Build history of the part. All positions in model axes, mm. A direction names the side the tool comes from. Give positions to 0.01 mm unless a question says otherwise; leave off trailing zeros. Write each loop counter-clockwise with the first axis right and the second up, starting at its lowest first coordinate (ties: lowest second). Pieces come first, ordered by that corner, then holes. Notation, with made-up numbers: (61, -17.5) -> (70, -17.5) arc R13 ccw to (70, -13.5) -> close; hole circle Ø5 at (18.25, 74). An arc over 180 degrees is marked (long way). One line per question, with ' | ' between items. Start each with the question number.
(1) Band-saw the part on B-B, the plane z = -41.5. Give the cut face in (x, y), and give its area (3 significant figures).
(2) Band-saw the part on C-C, the plane z = 10. Give the cut face in (x, y), and give its area (3 significant figures).
(3) Pin check, flat tips, straight feed: P1, Ø16, axis at x = -3, z = -45.5, coming from the -Y side; P2, Ø5, axis at y = -23.5, z = -55.5, coming from the +X side; P3, Ø7.5, axis at x = 17, y = -2, coming from the +Z side. Stop position of each tip, or through.
(4) Pull direction Y, two halves, no side cores. Call faces 6 (the flat face through (-16.26, 24.39, -4.52)), 7 (the cylindrical face through (-21.63, -19.44, -57.82)), 8 (the flat face through (-18.6, -20.2, -6)): released by +Y, released by -Y, zero draft, split by the parting line, or undercut.
(5) Tool access for faces 1 (the flat face through (-24.31, -16.18, -4.52)), 2 (the flat face through (16.26, -24.39, -4.52)), 3 (the flat face through (-24.11, 24.13, -50.4)), 4 (the flat face through (18, 17, -61)), 5 (the flat face through (-18, 0, 0)): list every direction of +Z, -Z, +X, -X, +Y, -Y with a clear straight run to the whole face (end or side of a thin tool).
(6) Drill centre lines: probe 1 along Y at (x, z) = (-20, -3.5); probe 2 along X at (y, z) = (0, -4.5); probe 3 along X at (y, z) = (11.5, -37.5). Where is each one in solid material? Low to high. Write a range as from..to.
(7) Band-saw the part on A-A, the plane y = 0. Give the cut face in (x, z), and give its area (3 significant figures).
from build123d import *
from build123d.topology import SkipClean

# Parameters (mm, degrees)
SKETCH1_R           = 2
BOSS_EXTRUDE1_DEPTH = 6
SKETCH2_R           = 25
SKETCH2_R_2         = 6.5
BOSS_EXTRUDE2_DEPTH = 2.5
SKETCH1_3_R         = 4
BOSS_EXTRUDE3_DEPTH = 30
CUT_EXTRUDE1_DEPTH  = 3
BOSS_EXTRUDE4_START = 34
SKETCH5_R           = 25.25
BOSS_EXTRUDE4_DEPTH = 34
BOSS_EXTRUDE5_START = 21
BOSS_EXTRUDE5_DEPTH = 21
BOSS_EXTRUDE6_START = 35.5
SKETCH7_R           = 25.25
BOSS_EXTRUDE6_DEPTH = 35.5
SKETCH8_R           = 7.5
BOSS_EXTRUDE7_DEPTH = 10
CIRPATTERN1_COUNT   = 4


with BuildPart() as part:
    # Sketch1 → Boss-Extrude1 (new body)
    with BuildSketch(Plane.XY):
        Polygon((-21.5, 27.25), (21.5, 27.25), (27.25, 21.5), (27.25, -21.5), (21.5, -27.25), (-21.5, -27.25), (-27.25, -21.5), (-27.25, 21.5), align=None)
        with Locations((20.859650045, 20.859650045)):
            Circle(SKETCH1_R, mode=Mode.SUBTRACT)
        with Locations((-20.859650045, 20.859650045)):
            Circle(SKETCH1_R, mode=Mode.SUBTRACT)
        with Locations((-20.859650045, -20.859650045)):
            Circle(SKETCH1_R, mode=Mode.SUBTRACT)
        with Locations((20.859650045, -20.859650045)):
            Circle(SKETCH1_R, mode=Mode.SUBTRACT)
    extrude(amount=-BOSS_EXTRUDE1_DEPTH)

    # Sketch2 → Boss-Extrude2 (add)
    with BuildSketch(Plane.XY):
        Circle(SKETCH2_R)
        Circle(SKETCH2_R_2, mode=Mode.SUBTRACT)
        with BuildLine():
            Line((-17.889167375, 13.646526688), (-13.234375729, 8.991735042))
            ThreePointArc((-13.234375729, 8.991735042), (-16, 0), (-13.234375729, -8.991735042))
            Line((-13.234375729, -8.991735042), (-17.889167375, -13.646526688))
            ThreePointArc((-17.889167375, -13.646526688), (-22.5, 0), (-17.889167375, 13.646526688))
        make_face(mode=Mode.SUBTRACT)
        with BuildLine():
            Line((-13.646526688, 17.889167375), (-8.991735042, 13.234375729))
            ThreePointArc((-8.991735042, 13.234375729), (0, 16), (8.991735042, 13.234375729))
            Line((8.991735042, 13.234375729), (13.646526688, 17.889167375))
            ThreePointArc((13.646526688, 17.889167375), (0, 22.5), (-13.646526688, 17.889167375))
        make_face(mode=Mode.SUBTRACT)
        with BuildLine():
            Line((17.889167375, 13.646526688), (13.234375729, 8.991735042))
            ThreePointArc((13.234375729, 8.991735042), (16, 0), (13.234375729, -8.991735042))
            Line((13.234375729, -8.991735042), (17.889167375, -13.646526688))
            ThreePointArc((17.889167375, -13.646526688), (22.5, 0), (17.889167375, 13.646526688))
        make_face(mode=Mode.SUBTRACT)
        with BuildLine():
            Line((8.991735042, -13.234375729), (13.646526688, -17.889167375))
            ThreePointArc((13.646526688, -17.889167375), (0, -22.5), (-13.646526688, -17.889167375))
            Line((-13.646526688, -17.889167375), (-8.991735042, -13.234375729))
            ThreePointArc((-8.991735042, -13.234375729), (0, -16), (8.991735042, -13.234375729))
        make_face(mode=Mode.SUBTRACT)
    extrude(amount=BOSS_EXTRUDE2_DEPTH)

    # Sketch1_3 → Boss-Extrude3 (add)
    with BuildSketch(Plane.XY):
        Circle(SKETCH1_3_R)
    extrude(amount=BOSS_EXTRUDE3_DEPTH)

    # Sketch3 → Cut-Extrude1 (cut)
    with BuildSketch(Plane(origin=(0, 0, -6), x_dir=(-1, 0, 0), z_dir=(0, 0, -1))):
        with BuildLine():
            Line((19.118272016, 27.25), (13.319474659, 21.451202643))
            ThreePointArc((13.319474659, 21.451202643), (0, 25.25), (-13.319474659, 21.451202643))
            Line((-13.319474659, 21.451202643), (-19.118272016, 27.25))
            Line((-19.118272016, 27.25), (19.118272016, 27.25))
        make_face()
        with BuildLine():
            Line((27.25, 19.118272016), (21.451202643, 13.319474659))
            ThreePointArc((21.451202643, 13.319474659), (25.25, 0), (21.451202643, -13.319474659))
            Line((21.451202643, -13.319474659), (27.25, -19.118272016))
            Line((27.25, -19.118272016), (27.25, 19.118272016))
        make_face()
        with BuildLine():
            Line((-27.25, 19.118272016), (-21.451202643, 13.319474659))
            ThreePointArc((-21.451202643, 13.319474659), (-25.25, 0), (-21.451202643, -13.319474659))
            Line((-21.451202643, -13.319474659), (-27.25, -19.118272016))
            Line((-27.25, -19.118272016), (-27.25, 19.118272016))
        make_face()
        with BuildLine():
            Line((-19.118272016, -27.25), (-13.319474659, -21.451202643))
            ThreePointArc((-13.319474659, -21.451202643), (0, -25.25), (13.319474659, -21.451202643))
            Line((13.319474659, -21.451202643), (19.118272016, -27.25))
            Line((19.118272016, -27.25), (-19.118272016, -27.25))
        make_face()
    extrude(amount=-CUT_EXTRUDE1_DEPTH, mode=Mode.SUBTRACT)

    # Sketch5 → Boss-Extrude4 (add)
    with BuildSketch(Plane(origin=(0, 0, -6), x_dir=(-1, 0, 0), z_dir=(0, 0, -1)).offset(BOSS_EXTRUDE4_START)):
        Circle(SKETCH5_R)
    extrude(amount=-BOSS_EXTRUDE4_DEPTH)

    # Sketch6 → Boss-Extrude5 (add)
    with SkipClean():  # the faces are left unmerged after this step: merging them gives an invalid solid
        with BuildSketch(Plane(origin=(0, 0, -40), x_dir=(-1, 0, 0), z_dir=(0, 0, -1)).offset(BOSS_EXTRUDE5_START)):
            with BuildLine():
                Line((-10, 23.185394109), (10, 23.185394109))
                ThreePointArc((10, 23.185394109), (10.910387984, 22.77116453), (11.803656596, 22.321204962))
                Line((11.803656596, 22.321204962), (22.382531694, 11.686948915))
                ThreePointArc((22.382531694, 11.686948915), (25.25, 0), (22.382531694, -11.686948915))
                Line((22.382531694, -11.686948915), (11.803656596, -22.321204962))
                ThreePointArc((11.803656596, -22.321204962), (10.910387984, -22.77116453), (10, -23.185394109))
                Line((10, -23.185394109), (-10, -23.185394109))
                ThreePointArc((-10, -23.185394109), (-10.910387984, -22.77116453), (-11.803656596, -22.321204962))
                Line((-11.803656596, -22.321204962), (-22.382531694, -11.686948915))
                ThreePointArc((-22.382531694, -11.686948915), (-25.25, 0), (-22.382531694, 11.686948915))
                Line((-22.382531694, 11.686948915), (-11.803656596, 22.321204962))
                ThreePointArc((-11.803656596, 22.321204962), (-10.910387984, 22.77116453), (-10, 23.185394109))
            make_face()
        extrude(amount=-BOSS_EXTRUDE5_DEPTH)

    # Sketch7 → Boss-Extrude6 (add)
    with SkipClean():  # the faces are left unmerged after this step: merging them gives an invalid solid
        with BuildSketch(Plane(origin=(0, 0, -61), x_dir=(-1, 0, 0), z_dir=(0, 0, -1)).offset(BOSS_EXTRUDE6_START)):
            Circle(SKETCH7_R)
        extrude(amount=-BOSS_EXTRUDE6_DEPTH)

    # Sketch8 → Boss-Extrude7 (add)
    with SkipClean():  # the faces are left unmerged after this step: merging them gives an invalid solid
        with BuildSketch(Plane(origin=(-17.093094145, 17.004076939, 0), x_dir=(0.7052583398611622, 0.7089504031004409, 0), z_dir=(-0.7089504031004409, 0.7052583398611622, 0))):
            with Locations(Location((0, 50.5, 0), (0, 0, 180))):
                Circle(SKETCH8_R)
        boss_extrude7 = extrude(amount=BOSS_EXTRUDE7_DEPTH)

    # CirPattern1: Boss-Extrude7 ×4 about axis
    with SkipClean():  # the faces are left unmerged after this step: merging them gives an invalid solid
        cirpattern1_axis = Axis((0, 0, 0), (0, 0, 1))
        for i in range(1, CIRPATTERN1_COUNT):
            add(boss_extrude7.rotate(cirpattern1_axis, i * 360 / CIRPATTERN1_COUNT))


solid = part.part
Results:
1) outline: (-22.38, -11.69) -> (-11.8, -22.32) arc R25.25 ccw to (-10, -23.19) -> (10, -23.19) arc R25.25 ccw to (11.8, -22.32) -> (22.38, -11.69) arc R25.25 ccw to (22.38, 11.69) -> (11.8, 22.32) arc R25.25 ccw to (10, 23.19) -> (-10, 23.19) arc R25.25 ccw to (-11.8, 22.32) -> (-22.38, 11.69) arc R25.25 ccw to start | area: 1,900 mm²
2) outline: circle Ø8 at (0, 0) | area: 50.3 mm²
3) P1: stops at y = -25.25 | P2: stops at x = 27.22 | P3: stops at z = 2.5
4) face 6: released by +Y | face 7: undercut | face 8: zero draft
5) face 1: -X | face 2: -Y | face 3: -Z, -X, +Y | face 4: +X, +Y | face 5: +Z
6) probe 1: y = -27.25..-22.67, -19.05..19.05, 22.67..27.25 | probe 2: x = -25.25..25.25 | probe 3: x = -22.48..22.48
7) outline: (-27.25, -3) -> (-25.25, -3) -> (-25.25, -96.5) -> (25.25, -96.5) -> (25.25, -3) -> (27.25, -3) -> (27.25, 0) -> (25, 0) -> (25, 2.5) -> (22.5, 2.5) -> (22.5, 0) -> (16, 0) -> (16, 2.5) -> (6.5, 2.5) -> (6.5, 0) -> (4, 0) -> (4, 30) -> (-4, 30) -> (-4, 0) -> (-6.5, 0) -> (-6.5, 2.5) -> (-16, 2.5) -> (-16, 0) -> (-22.5, 0) -> (-22.5, 2.5) -> (-25, 2.5) -> (-25, 0) -> (-27.25, 0) -> close | area: 5,190 mm²
